```python
from build123d import *

# Parameters (mm, degrees)
SKETCH2_W           = 254
SKETCH2_H           = 165.1
BOSS_EXTRUDE1_DEPTH = 6.35
SKETCH3_W           = 241.3
SKETCH3_H           = 152.4
BOSS_EXTRUDE2_DEPTH = 6.35
SKETCH4_R           = 20.32
CUT_EXTRUDE2_DEPTH  = 153.002606886


with BuildPart() as part:
    # Sketch2 → Boss-Extrude1 (new body)
    with BuildSketch(Plane(origin=(0, 0, 0), x_dir=(1, 0, 0), z_dir=(0, 1, 0))):
        Rectangle(SKETCH2_W, SKETCH2_H)
    extrude(amount=BOSS_EXTRUDE1_DEPTH)

    # Sketch3 → Boss-Extrude2 (add)
    with BuildSketch(Plane(origin=(0, 6.35, 0), x_dir=(1, 0, 0), z_dir=(0, 1, 0))):
        Rectangle(SKETCH3_W, SKETCH3_H)
    extrude(amount=BOSS_EXTRUDE2_DEPTH)

    # Sketch4 → Cut-Extrude2 (cut, through all)
    with BuildSketch(Plane(origin=(0, 12.7, 0), x_dir=(1, 0, 0), z_dir=(0, 1, 0))):
        with Locations(Location((-60.325, 38.1, 0), (0, 0, 270))):
            Circle(SKETCH4_R)
        with Locations(Location((60.325, 38.1, 0), (0, 0, 90))):
            Circle(SKETCH4_R)
        with Locations(Location((60.325, -38.1, 0), (0, 0, 270))):
            Circle(SKETCH4_R)
        with Locations(Location((-60.325, -38.1, 0), (0, 0, 90))):
            Circle(SKETCH4_R)
    extrude(amount=-CUT_EXTRUDE2_DEPTH, mode=Mode.SUBTRACT)


solid = part.part
```
Work out the finished part from the listing and answer in its coordinate system (mm). A direction names the side the tool comes from. Coordinates: 2 decimals unless noted, no trailing zeros. Write each loop counter-clockwise with the first axis right and the second up, starting at its lowest first coordinate (ties: lowest second). Pieces come first, ordered by that corner, then holes. Notation, with made-up numbers: (81.5, 66) - (122.5, 66) arc R15 cw to (122.5, 95) - close; hole circle Ø7 at (-28.5, 81). An arc over 180 degrees is marked (long way). Answer as a JSON object with one key per item and string values.
Q1. For a pull along Z with two mould halves and no side action, classify faces 4 (the flat face through (-120.65, 9, 1)), 5 (the cylindrical face through (-54.22, 6.44, -18.72)), 6 (the flat face through (-2, 9, 76.2)) as pulls with the +Z half, pulls with the -Z half, needs draft (parallel to the pull), parting line crosses it, or undercut.
Results list:
{"face 4": "needs draft", "face 5": "undercut", "face 6": "pulls with the +Z half"}
Q2. Find section A-A (z = -38.1). Write down the section's boundary in (x, y) (3 decimals).
Results list:
{"outline": "(-127, 0) - (-80.645, 0) - (-80.645, 12.7) - (-120.65, 12.7) - (-120.65, 6.35) - (-127, 6.35) - close; (-40.005, 0) - (40.005, 0) - (40.005, 12.7) - (-40.005, 12.7) - close; (80.645, 0) - (127, 0) - (127, 6.35) - (120.65, 6.35) - (120.65, 12.7) - (80.645, 12.7) - close"}
Q3. Which of the six approach directions +Z, -Z, +X, -X, +Y, -Y give full straight-line access (tool end or side, diameter ignored) to faces 1 (the flat face through (-2, 9, -76.2)), 2 (the flat face through (120.65, 9, 1)), 3 (the flat face through (-127, 3, 1))?
Results list:
{"face 1": "-Z, +X, -X, +Y", "face 2": "+Z, -Z, +X, +Y", "face 3": "+Z, -Z, -X, +Y, -Y"}
Q4. Find section D-D (x = 15). Write down the section's boundary in (y, z), plus the area to 3 significant figures.
Results list:
{"outline": "(0, -82.55) - (6.35, -82.55) - (6.35, -76.2) - (12.7, -76.2) - (12.7, 76.2) - (6.35, 76.2) - (6.35, 82.55) - (0, 82.55) - close", "area": "2,020 mm^2"}
Q5. Given pin 1 Ø3 at (y, z) = (9, 8.5) entering from +X; pin 2 Ø1.9 at (x, y) = (-1.5, 10) entering from +Z; pin 3 Ø3 at (y, z) = (11, -36) entering from -X, each flat-ended and moving along its own axis, determine where each tip first touches the part or whether it passes through.
Results list:
{"pin 1": "stops at x = 120.65", "pin 2": "stops at z = 76.2", "pin 3": "stops at x = -120.65"}
Q6. Find section C-C (x = -65). Write down the section's boundary in (y, z).
Results list:
{"outline": "(0, -82.55) - (6.35, -82.55) - (6.35, -76.2) - (12.7, -76.2) - (12.7, -57.87) - (0, -57.87) - close; (0, -18.33) - (12.7, -18.33) - (12.7, 18.33) - (0, 18.33) - close; (0, 57.87) - (12.7, 57.87) - (12.7, 76.2) - (6.35, 76.2) - (6.35, 82.55) - (0, 82.55) - close"}
Q7. Consider L1, parallel to X at y = 9.75, z = 38.1 (3 decimals); L2, parallel to X at y = 3.5, z = 38.1 (3 decimals); L3, parallel to Z at x = -53, y = 8. Determine where each line is inside the solid, lowest interval first. Write a range as from..to.
Results list:
{"L1": "x = -120.65..-80.645, -40.005..40.005, 80.645..120.65", "L2": "x = -127..-80.645, -40.005..40.005, 80.645..127", "L3": "z = -76.2..-57.05, -19.15..19.15, 57.05..76.2"}
Q8. Find section B-B (y = 8.75). Write down the section's boundary in (x, z) (3 decimals).
Results list:
{"outline": "(-120.65, -76.2) - (120.65, -76.2) - (120.65, 76.2) - (-120.65, 76.2) - close; hole circle Ø40.64 at (-60.325, -38.1); hole circle Ø40.64 at (-60.325, 38.1); hole circle Ø40.64 at (60.325, -38.1); hole circle Ø40.64 at (60.325, 38.1)"}
